from build123d import *

# Parameters (mm, degrees)
SKETCH1_W           = 20
SKETCH1_H           = 20
BOSS_EXTRUDE1_DEPTH = 20
CUT_EXTRUDE1_DEPTH  = 20
CUT_EXTRUDE2_DEPTH  = 20
CUT_EXTRUDE3_DEPTH  = 20


with BuildPart() as part:
    # Sketch1 → Boss-Extrude1 (new body)
    with BuildSketch(Plane.XY):
        with Locations((10, 10)):
            Rectangle(SKETCH1_W, SKETCH1_H)
    extrude(amount=BOSS_EXTRUDE1_DEPTH)

    # Sketch2 → Cut-Extrude1 (cut)
    with BuildSketch(Plane(origin=(0, 20, 0), x_dir=(1, 0, 0), z_dir=(0, 1, 0))):
        Polygon((0, 0), (20, 0), (20, -10), align=None)
    extrude(amount=-CUT_EXTRUDE1_DEPTH, mode=Mode.SUBTRACT)

    # Sketch3 → Cut-Extrude2 (cut)
    with BuildSketch(Plane(origin=(0, 20, 0), x_dir=(1, 0, 0), z_dir=(0, 1, 0))):
        Polygon((0, 0), (0, -20), (10, -20), align=None)
    extrude(amount=-CUT_EXTRUDE2_DEPTH, mode=Mode.SUBTRACT)

    # Sketch4 → Cut-Extrude3 (cut)
    with BuildSketch(Plane(origin=(0, 20, 0), x_dir=(1, 0, 0), z_dir=(0, 1, 0))):
        Polygon((20, -20), (20, -10), (10, -20), align=None)
    extrude(amount=-CUT_EXTRUDE3_DEPTH, mode=Mode.SUBTRACT)


solid = part.part
Design review of the part built by this model. Coordinates are the model's own, in mm. Coordinates: 2 decimals unless noted, no trailing zeros. Loops run counter-clockwise (first coordinate to the right, second up) from the corner with the lowest first, then second, coordinate; pieces in that order, holes last.
Item 1: Add section C-C (x = 1.5). Write out the cut boundary in (y, z), and give its area (3 significant figures).
Completed:
outline: (0, 0.75) - (20, 0.75) - (20, 3) - (0, 3) - close
area: 45.0 mm2
Item 2: Clearance check with flat-ended pins moving along their axes: pin 1 (2 mm diameter, centred on x = 16.5, y = 15.5, fed in from -Z); pin 2 (3 mm diameter, centred on x = 15, y = 8, fed in from +Z); pin 3 (3 mm diameter, centred on y = 12.5, z = 3.5, fed in from -X); pin 4 (3 mm diameter, centred on x = 3.5, z = 4.5, fed in from -Y). State where each tip first meets the part, or that it passes through.
Completed:
pin 1: stops at z = 7.75
pin 2: stops at z = 16.5
pin 3: stops at x = 1
pin 4: stops at y = 0
Item 3: Add section A-A (y = 11.75). Write out the cut boundary in (x, z).
Completed:
outline: (0, 0) - (20, 10) - (10, 20) - close
Item 4: Add section B-B (z = 5). Write out the cut boundary in (x, y).
Completed:
outline: (2.5, 0) - (10, 0) - (10, 20) - (2.5, 20) - close
Item 5: Wall thickness on L1, parallel to X at y = 2.25, z = 2; L2, parallel to Z at x = 9.75, y = 16 (3 decimals); L3, parallel to X at y = 1.75, z = 16.75 (3 decimals): over which ranges is each line inside the solid? List them lowest first.
Completed:
L1: x = 1 to 4
L2: z = 4.875 to 19.5
L3: x = 8.375 to 13.25
